Here's how the part is built. I have some questions about the finished solid (model axes, mm). Face numbers are marked on the shaded views. A direction names the side the tool comes from. Give positions to 0.01 mm unless a question says otherwise; leave off trailing zeros. Write each loop counter-clockwise with the first axis right and the second up, starting at its lowest first coordinate (ties: lowest second). Pieces come first, ordered by that corner, then holes. Notation, with made-up numbers: (13, -12.5) -> (63, -12.5) arc R13 cw to (63, 12.5) -> close; hole circle Ø7 at (-25.5, 46.5). An arc over 180 degrees is marked (long way). Put each result on its own line as item: value. Start each with the question number.
from build123d import *

# Parameters (mm, degrees)
F0_R     = 19.05
F1_DEPTH = 25.4


with BuildPart() as f1:
    # F0 (on Front) → F1 (new body)
    with BuildSketch(Plane.XZ):
        with BuildLine():
            ThreePointArc((-76.2, 208.182272), (-147.207096, 36.755978), (0, -76.2))
            ThreePointArc((0, -76.2), (76.2, 0), (0, 76.2))
            ThreePointArc((0, 76.2), (-34.697045, 85.497045), (-25.4, 120.194091))
            ThreePointArc((-25.4, 120.194091), (-6.805909, 189.588181), (-76.2, 208.182272))
        make_face()
        Circle(F0_R, mode=Mode.SUBTRACT)
        with BuildLine():
            ThreePointArc((-60.325, 180.685965), (-41.275, 180.685965), (-31.75, 164.188181))
            ThreePointArc((-31.75, 164.188181), (-34.302216, 154.663181), (-41.275, 147.690397))
            ThreePointArc((-41.275, 147.690397), (-79.737177, 97.565512), (-71.490397, 34.925))
            ThreePointArc((-71.490397, 34.925), (-69.587294, 30.330503), (-68.938181, 25.4))
            ThreePointArc((-68.938181, 25.4), (-83.057678, 6.999113), (-104.485965, 15.875))
            ThreePointArc((-104.485965, 15.875), (-116.538951, 107.426518), (-60.325, 180.685965))
        make_face(mode=Mode.SUBTRACT)
    extrude(amount=F1_DEPTH)


solid = f1.part
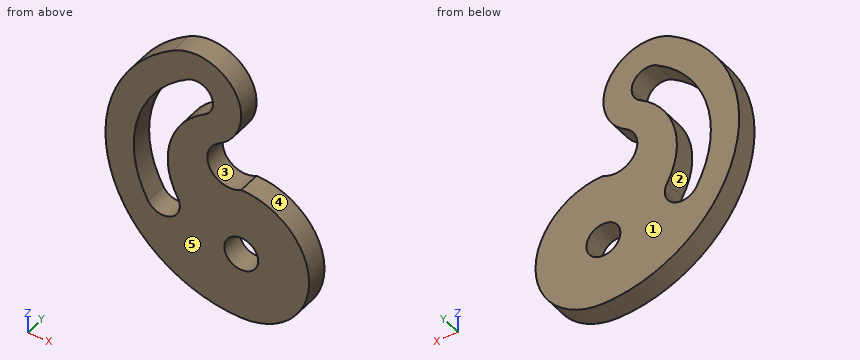
1) I'm going to push flat-ended pins straight in: pin 1 Ø5 at (x, z) = (17.5, 6) entering from +Y; pin 2 Ø4 at (y, z) = (-3.5, 185.5) entering from +X; pin 3 Ø4 at (x, y) = (-80, -8.5) entering from -Z; pin 4 Ø1 at (y, z) = (-9, -45) entering from -X. Where does each tip first touch, or does it pass through?
2) I need wall thicknesses on probe 1 along Z at (x, y) = (10, -23.25); probe 2 along X at (y, z) = (-3, -11); probe 3 along X at (y, z) = (-8.5, 97.5). Which ranges of each line are inside material? Lowest first, please.
3) I want a section at B-B, the plane z = 0. Write out the boundary of the cut face in (x, y).
4) Thinking about a two-plate mould opening in Z: for the marked faces 3, 4 and 5, which applies, released by +Z, released by -Z, zero draft, split by the parting line, or undercut?
5) I want a section at D-D, the plane x = -89.5. Write out the boundary of the cut face in (y, z).
6) I want a section at A-A, the plane y = -10. Write out the boundary of the cut face in (x, z) (3 decimals).
7) I want a section at C-C, the plane x = -12.7. Write out the boundary of the cut face in (y, z).
8) Which directions (+Z, -Z, +X, -X, +Y, -Y) give clear straight access to the entire face, cutting with the end or side of a thin tool? Please do the marked faces 1 and 2.
Established:
1. pin 1: stops at y = 0
1. pin 2: stops at x = -3.81
1. pin 3: stops at z = -54.73
1. pin 4: stops at x = -93.04
2. probe 1: z = -75.54 to -16.21, 16.21 to 75.54
2. probe 2: x = -124.99 to -15.55, 15.55 to 75.4
2. probe 3: x = -150.9 to -118.75, -79.75 to -38.09
3. outline: (-131.98, -25.4) -> (-19.05, -25.4) -> (-19.05, 0) -> (-131.98, 0) -> close; (19.05, -25.4) -> (76.2, -25.4) -> (76.2, 0) -> (19.05, 0) -> close
4. face 3: undercut
4. face 4: split by the parting line
4. face 5: zero draft
5. outline: (-25.4, -47.15) -> (0, -47.15) -> (0, 6.41) -> (-25.4, 6.41) -> close; (-25.4, 157.11) -> (0, 157.11) -> (0, 199.55) -> (-25.4, 199.55) -> close
6. outline: (-76.2, 208.182) arc R152.4 ccw to (0, -76.2) arc R76.2 ccw to (0, 76.2) arc R25.4 cw to (-25.4, 120.194) arc R50.8 ccw to start; hole (-104.486, 15.875) arc R19.05 ccw to (-71.49, 34.925) arc R82.55 cw to (-41.275, 147.69) arc R19.05 ccw to (-60.325, 180.686) arc R120.65 ccw to start; hole circle Ø38.1 at (0, 0)
7. outline: (-25.4, -75.67) -> (0, -75.67) -> (0, -14.2) -> (-25.4, -14.2) -> close; (-25.4, 14.2) -> (0, 14.2) -> (0, 72.8) -> (-25.4, 72.8) -> close; (-25.4, 130.59) -> (0, 130.59) -> (0, 197.79) -> (-25.4, 197.79) -> close
8. face 1: +Z, -Z, +X, -X, +Y
8. face 2: +Y, -Y
